```python
from build123d import *

# Parameters (mm, degrees)
SKETCH1_R             = 3.45
SKETCH1_R_2           = 1.45
BOSS_EXTRUDE1_DEPTH   = 8.5
BOSS_EXTRUDE1_2_DEPTH = 8.5
BOSS_EXTRUDE1_3_DEPTH = 8.5
SKETCH2_R             = 1.45
BOSS_EXTRUDE2_DEPTH   = 2
FILLET2_R             = 2.5


with BuildPart() as part:
    # Sketch1 → Boss-Extrude1 (new body)
    with BuildSketch(Plane(origin=(0, 0, 0), x_dir=(1, 0, 0), z_dir=(0, 1, 0))):
        with Locations(Location((-52.25, 5, 0), (0, 0, 270))):
            Circle(SKETCH1_R)
        with Locations(Location((-52.25, 5, 0), (0, 0, 270))):
            Circle(SKETCH1_R_2, mode=Mode.SUBTRACT)
    extrude(amount=BOSS_EXTRUDE1_DEPTH)



with BuildPart() as body_2:
    # Sketch1 → Boss-Extrude1 2 (new body)
    with BuildSketch(Plane(origin=(0, 0, 0), x_dir=(1, 0, 0), z_dir=(0, 1, 0))):
        with Locations(Location((0, 0, 0), (0, 0, 270))):
            Circle(SKETCH1_R)
        with Locations(Location((0, 0, 0), (0, 0, 270))):
            Circle(SKETCH1_R_2, mode=Mode.SUBTRACT)
    extrude(amount=BOSS_EXTRUDE1_2_DEPTH)


with BuildPart() as body_3:
    # Sketch1 → Boss-Extrude1 3 (new body)
    with BuildSketch(Plane(origin=(0, 0, 0), x_dir=(1, 0, 0), z_dir=(0, 1, 0))):
        with Locations(Location((0, -28, 0), (0, 0, 270))):
            Circle(SKETCH1_R)
        with Locations(Location((0, -28, 0), (0, 0, 270))):
            Circle(SKETCH1_R_2, mode=Mode.SUBTRACT)
    extrude(amount=BOSS_EXTRUDE1_3_DEPTH)


with BuildPart() as part_1:
    add(part.part)

    add(body_2.part)  # Boss-Extrude2 merges body 2

    add(body_3.part)  # Boss-Extrude2 merges body 3
    # Sketch2 → Boss-Extrude2 (add)
    with BuildSketch(Plane(origin=(0, 0, 0), x_dir=(1, 0, 0), z_dir=(0, 1, 0))):
        Polygon((5, 5), (5, -33), (-5, -33), (-57.25, 0), (-57.25, 10), (-47.25, 10), (-47.25, 5), align=None)
        with Locations(Location((-52.25, 5, 0), (0, 0, 270))):
            Circle(SKETCH2_R, mode=Mode.SUBTRACT)
        with Locations(Location((0, -28, 0), (0, 0, 270))):
            Circle(SKETCH2_R, mode=Mode.SUBTRACT)
        with Locations(Location((0, 0, 0), (0, 0, 270))):
            Circle(SKETCH2_R, mode=Mode.SUBTRACT)
        Polygon((-33.5, -5), (-5, -23), (-5, -5), align=None, mode=Mode.SUBTRACT)
    extrude(amount=BOSS_EXTRUDE2_DEPTH)

    # Fillet2
    fillet2_edges = [part_1.edges().sort_by_distance(p)[0] for p in [
        (-5, 1, 33),
        (-57.25, 1, 0),
        (-57.25, 1, -10),
        (-47.25, 1, -5),
        (5, 1, -5),
        (5, 1, 33),
        (-47.25, 1, -10),
        (-33.5, 1, 5),
        (-5, 1, 5),
        (-5, 1, 23),
    ]]
    fillet(fillet2_edges, radius=FILLET2_R - 0.0001)  # a hair under: the kernel refuses the full size


with BuildPart() as body_2_2:
    # Mirror1: mirrored copy
    add(part_1.part.mirror(Plane.XY))


solid = body_2_2.part
```
Work out the finished part from the listing and answer in its coordinate system (mm). A direction names the side the tool comes from. Round coordinates to 2 decimals unless told otherwise and drop trailing zeros. Write each loop counter-clockwise with the first axis right and the second up, starting at its lowest first coordinate (ties: lowest second). Pieces come first, ordered by that corner, then holes.
1) Consider probe 1 along X at (y, z) = (3.75, 5); probe 2 along X at (y, z) = (5, -28); probe 3 along Y at (x, z) = (-4, -10.5). Determine where each line is inside the solid, lowest interval first.
2) A cutting plane is placed at D-D on x = -19. Determine the outline of the cut face in (y, z).
3) Flat-ended cylindrical pins translate along their axes: P1, Ø0.6, axis at x = -29, y = 0.5, coming from the +Z side; P2, Ø21.5, axis at x = -18, z = -7.5, coming from the +Y side; P3, Ø1.6, axis at x = -12.5, y = 1, coming from the -Z side. Find the tip coordinate at first contact, or state that the pin passes through.
4) A cutting plane is placed at B-B on z = -13.5. Determine the outline of the cut face in (x, y) (3 decimals).
5) Which of the six approach directions +Z, -Z, +X, -X, +Y, -Y give full straight-line access (tool end or side, diameter ignored) to faces 1 (the face through (-55.618, 5.204, 5.748)), 2 (the face through (-17.637, 0.986, -15.019)), 3 (the face through (-21, 1, 5)), 4 (the face through (-0.7, 8.5, -29.5))?
6) A cutting plane is placed at C-C on x = 0. Determine the outline of the cut face in (y, z), and give its area (3 significant figures).
7) A cutting plane is placed at A-A on y = 4.75. Determine the outline of the cut face in (x, z), and give its area (3 significant figures).
Entries:
1. probe 1: x = -55.7 to -53.7, -50.8 to -48.8
1. probe 2: x = -3.45 to -1.45, 1.45 to 3.45
1. probe 3: y = 0 to 2
2. outline: (0, -24.16) - (2, -24.16) - (2, -14.16) - (0, -14.16) - close; (0, -5) - (2, -5) - (2, 5) - (0, 5) - close
3. P1: stops at z = 5
3. P2: stops at y = 2
3. P3: stops at z = -28.77
4. outline: (-35.875, 0) - (-20.042, 0) - (-20.042, 2) - (-35.875, 2) - close; (-5, 0) - (5, 0) - (5, 2) - (-5, 2) - close
5. face 1: +Y
5. face 2: +Y, -Y
5. face 3: +Z, +X, +Y, -Y
5. face 4: +Z, -Z, +X, -X, +Y
6. outline: (0, -33) - (2, -33) - (2, -31.45) - (8.5, -31.45) - (8.5, -29.45) - (0, -29.45) - close; (0, -26.55) - (8.5, -26.55) - (8.5, -24.55) - (2, -24.55) - (2, -3.45) - (8.5, -3.45) - (8.5, -1.45) - (0, -1.45) - close; (0, 1.45) - (8.5, 1.45) - (8.5, 3.45) - (2, 3.45) - (2, 5) - (0, 5) - close
6. area: 116 mm2
7. outline: circle Ø6.9 at (-52.25, 5); circle Ø6.9 at (0, -28); circle Ø6.9 at (0, 0); hole circle Ø2.9 at (-52.25, 5); hole circle Ø2.9 at (0, -28); hole circle Ø2.9 at (0, 0)
7. area: 92.4 mm2
